Can you work these out from the model? Positions are in its coordinate system, mm. Face numbers are marked on the shaded views. A direction names the side the tool comes from. Round coordinates to 2 decimals unless told otherwise and drop trailing zeros. Loops run counter-clockwise (first coordinate to the right, second up) from the corner with the lowest first, then second, coordinate; pieces in that order, holes last. Notation, with made-up numbers: (2, 43) -> (54, 43) arc R10 cw to (54, 54) -> close; hole circle Ø5 at (82, 57). An arc over 180 degrees is marked (long way). Write item = value, one per line.
from build123d import *

# Parameters (mm, degrees)
F0_W     = 1000
F0_H     = 300
F0_W_2   = 960
F0_H_2   = 260
F1_DEPTH = 100
F3_DEPTH = 100
F4_W     = 1000
F4_H     = 300
F4_W_2   = 960
F4_H_2   = 260
F5_DEPTH = 100


with BuildPart() as f1:
    # F0 (on Front) → F1 (new body)
    with BuildSketch(Plane.XZ):
        with Locations((500, 150)):
            Rectangle(F0_W, F0_H)
        with Locations((500, 150)):
            Rectangle(F0_W_2, F0_H_2, mode=Mode.SUBTRACT)
    extrude(amount=F1_DEPTH)

    # F2 (on Front) → F3 (join)
    with BuildSketch(Plane.XZ):
        Polygon((0, 225), (0, 75), (75, 0), (925, 0), (1000, 75), (1000, 225), (925, 300), (75, 300), align=None)
        Polygon((20, 83.284271), (20, 216.715729), (83.284271, 280), (916.715729, 280), (980, 216.715729), (980, 83.284271), (916.715729, 20), (83.284271, 20), align=None, mode=Mode.SUBTRACT)
    extrude(amount=-F3_DEPTH)

    # F4 (on face) → F5 (join)
    with BuildSketch(Plane(origin=(0, 100, 0), x_dir=(-1, 0, 0), z_dir=(0, 1, 0))):
        with Locations((-500, 150)):
            Rectangle(F4_W, F4_H)
        with Locations((-500, 150)):
            Rectangle(F4_W_2, F4_H_2, mode=Mode.SUBTRACT)
    extrude(amount=F5_DEPTH)


solid = f1.part
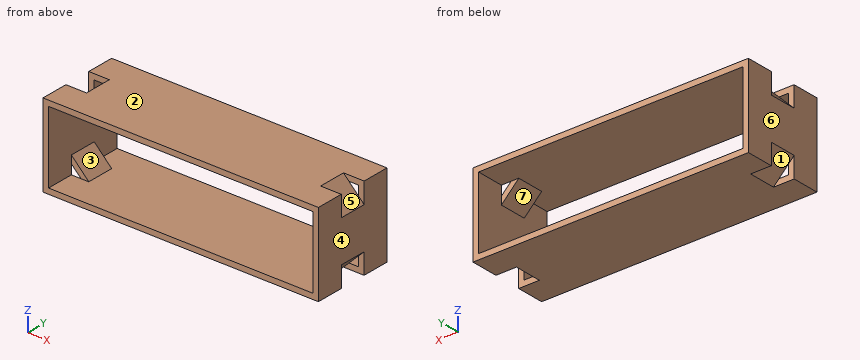
1. Suppose I cut it at A-A, the plane y = 78. List the corners of the cut face in (x, z) for me.
Entries:
outline = (0, 75) -> (75, 0) -> (925, 0) -> (1000, 75) -> (1000, 225) -> (925, 300) -> (75, 300) -> (0, 225) -> close; hole (20, 83.28) -> (83.28, 20) -> (916.72, 20) -> (980, 83.28) -> (980, 216.72) -> (916.72, 280) -> (83.28, 280) -> (20, 216.72) -> close
2. I need wall thicknesses on line 1 (X direction, y = -33, z = 24.5); line 2 (Z direction, x = 757, y = 126); line 3 (X direction, y = 96, z = 30). Which ranges of each line are inside material? Lowest first, please. Write a range as [from, to].
Entries:
line_1 = [0, 20], [980, 1000]
line_2 = [0, 20], [280, 300]
line_3 = [45, 73.28], [926.72, 955]
3. Suppose I cut it at B-B, the plane x = 335.5. List the corners of the cut face in (y, z) for me, and give its area (3 significant figures).
Entries:
outline = (-100, 0) -> (200, 0) -> (200, 20) -> (-100, 20) -> close; (-100, 280) -> (200, 280) -> (200, 300) -> (-100, 300) -> close
area = 12,000 mm²
4. I'm going to push a flat-ended pin straight in: pin 1 (2 mm diameter, centred on y = 80, z = 244, fed in from +X). Where does the tip first touch, or does it pass through?
Entries:
pin_1 = 982
5. Suppose I cut it at D-D, the plane z = 256. List the corners of the cut face in (x, y) for me, and give its area (3 significant figures).
Entries:
outline = (0, -100) -> (20, -100) -> (20, 0) -> (0, 0) -> close; (0, 100) -> (20, 100) -> (20, 200) -> (0, 200) -> close; (31, 0) -> (59.28, 0) -> (59.28, 100) -> (31, 100) -> close; (940.72, 0) -> (969, 0) -> (969, 100) -> (940.72, 100) -> close; (980, -100) -> (1000, -100) -> (1000, 0) -> (980, 0) -> close; (980, 100) -> (1000, 100) -> (1000, 200) -> (980, 200) -> close
area = 13,700 mm²
6. Suppose I cut it at C-C, the plane z = 148. List the corners of the cut face in (x, y) for me.
Entries:
outline = (0, -100) -> (20, -100) -> (20, 200) -> (0, 200) -> close; (980, -100) -> (1000, -100) -> (1000, 200) -> (980, 200) -> close
7. For the marked faces 5, 6 and 7, which set-ups out of +Z, -Z, +X, -X, +Y, -Y let a thin tool reach every point of the face, with its end or its side?
Entries:
face_5 = +Z, +X
face_6 = +Z, -Z, -X, +Y, -Y
face_7 = +Y, -Y
8. We'd pull the mould along Z, two halves only. Please class the marked faces 1, 2, 3 and 4: released by +Z, released by -Z, zero draft, split by the parting line, or undercut.
Entries:
face_1 = released by -Z
face_2 = released by +Z
face_3 = undercut
face_4 = zero draft
